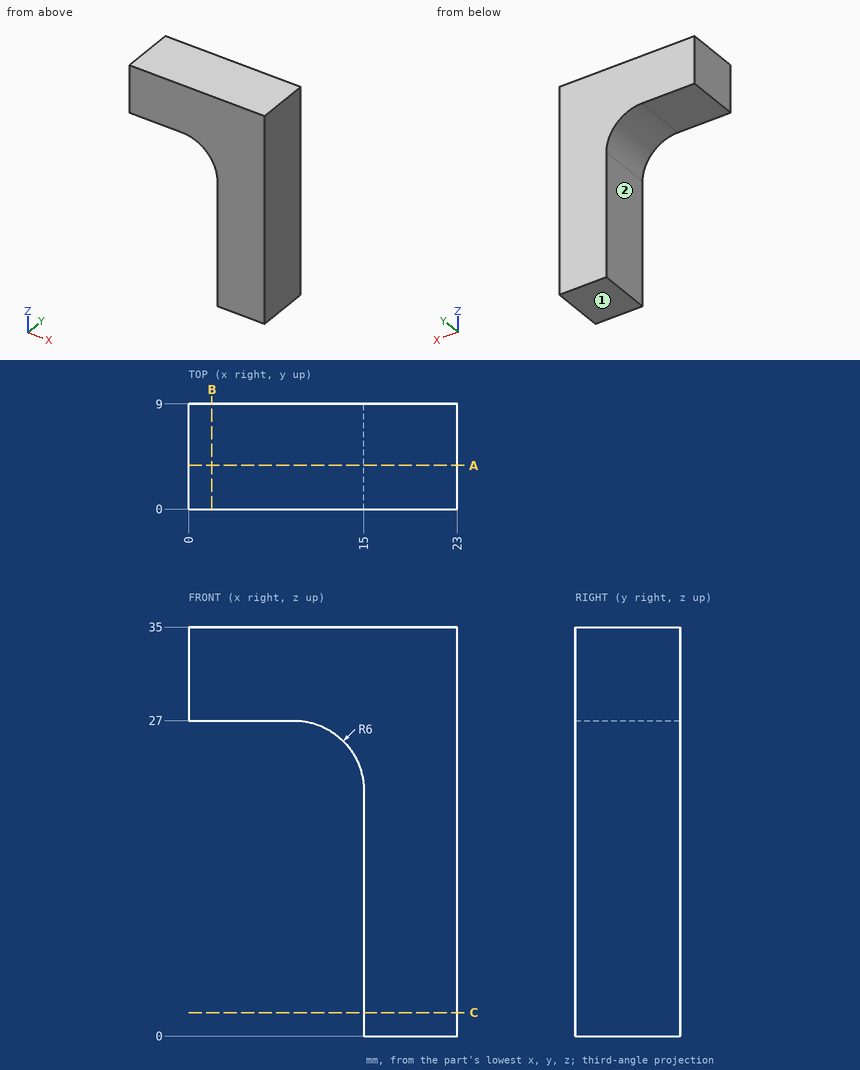
Here's the drawing with two shaded views (mm, measured from the low corner). I have some questions. A direction names the side the tool comes from. Round coordinates to 2 decimals unless told otherwise and drop trailing zeros. Loops run counter-clockwise (first coordinate to the right, second up) from the corner with the lowest first, then second, coordinate; pieces in that order, holes last.
1. If I drill on probe 1 along Z at (x, y) = (2.75, 2); probe 2 along X at (y, z) = (2.5, 9); probe 3 along Z at (x, y) = (10.75, 8.5), over which ranges is the centre line in solid material (lowest first)?
Answers:
probe 1: z = 27 to 35
probe 2: x = 15 to 23
probe 3: z = 26.74 to 35
2. Suppose I cut it at A-A, the plane y = 3.75. Please give me the cut outline in (x, z), and give its area (3 significant figures).
Answers:
outline: (0, 27) - (9, 27) arc R6 cw to (15, 21) - (15, 0) - (23, 0) - (23, 35) - (0, 35) - close
area: 408 mm2
3. Suppose I cut it at B-B, the plane x = 2. Please give me the cut outline in (y, z).
Answers:
outline: (0, 27) - (9, 27) - (9, 35) - (0, 35) - close
4. Suppose I cut it at C-C, the plane z = 2. Please give me the cut outline in (x, y).
Answers:
outline: (15, 0) - (23, 0) - (23, 9) - (15, 9) - close
5. For the marked faces 1 and 2, which set-ups out of +Z, -Z, +X, -X, +Y, -Y let a thin tool reach every point of the face, with its end or its side?
Answers:
face 1: -Z, +X, -X, +Y, -Y
face 2: -Z, -X, +Y, -Y
6. Will these pins go through, and if not, where does the flat tip stop? pin 1 (2 mm diameter, centred on y = 6.5, z = 24, fed in from -X); pin 2 (5 mm diameter, centred on x = 6, z = 23.5, fed in from -Y).
Answers:
pin 1: stops at x = 13.47
pin 2: passes through
